Here's how the part is built. I have some questions about the finished solid (model axes, mm). Face numbers are marked on the shaded views. A direction names the side the tool comes from. Round coordinates to 2 decimals unless told otherwise and drop trailing zeros. Order: outer loops, then holes, each group sorted by start corner. A loop starts at its lowest first (then second) coordinate and runs counter-clockwise, first axis right, second up. Notation, with made-up numbers: (66.5, 63.25) -> (107.5, 63.25) arc R26 ccw to (107.5, 101.25) -> close; hole circle Ø4 at (24, 47.5). An arc over 180 degrees is marked (long way). Answer in a Markdown table with one row per item.
Autodesk Inventor part; units mm, degrees
ref_plane "Płaszczyzna konstrukcyjna1" through (0, 0, 8) normal (0, 0, -1) x (-1, 0, 0)
ref_plane "YZ Plane" through (0, 0, 0) normal (1, 0, 0) x (0, 1, 0)
ref_plane "XZ Plane" through (0, 0, 0) normal (0, 1, 0) x (-1, 0, 0)
sketch "Szkic1" plane through (0, 0, 0) normal (0, 0, 1) x (1, 0, 0)
  line L0 (-14, 0) -> (14, 0)
  line L1 (0, -14) -> (0, 14)
  circle A0 centre (0, 0) radius 10
  circle A1 centre (0, 0) radius 1.8
  line L2 (-1.3416, 1.2) -> (1.3416, 1.2)
  dimension "d1" = 20
  dimension "d2" = 3.6
  dimension "d3" = 1.2
extrude "Wyciągnięcie proste1" add sketch "Szkic1" along normal blind 20 contours A1 L1 A0 L0 | L0 A0 L1 A1 | L2 L1 A1 | L1 A0 L0 A1 | L1 A1 L0 A0 | L2 A1 L1
ref_plane "Płaszczyzna konstrukcyjna1" through (0, 0, 8) normal (0, 0, -1) x (-1, 0, 0)
sketch "Szkic2" plane through (0, 0, 8) normal (0, 0, -1) x (-1, 0, 0)
  circle A0 centre (0, 0) radius 10
  arc A1 (-1.3416, 1.2) -> (1.3416, 1.2) centre (0, 0) ccw
  line L0 (1.3416, 1.2) -> (-1.3416, 1.2)
  circle A2 centre (0, 0) radius 12
  dimension "d7" = 24
extrude "Wyciągnięcie proste2" add sketch "Szkic2" against normal blind 4 contours A2
sketch "Szkic3" plane through (0, 0, 0) normal (0, 0, -1) x (-1, 0, 0)
  circle A0 centre (0, 0) radius 10
  arc A1 (-1.3416, 1.2) -> (1.3416, 1.2) centre (0, 0) ccw
  line L0 (1.3416, 1.2) -> (-1.3416, 1.2)
  circle A2 centre (0, 0) radius 12
  circle A3 centre (0, 0) radius 10
  line L1 (16.8, 0) -> (-16.8, 0)
  line L2 (0, -16.8) -> (0, 16.8)
  line L3 (2, -11) -> (-2, -11)
  line L4 (-2, -11) -> (-2, -9)
  line L5 (-2, -9) -> (2, -9)
  line L6 (2, -9) -> (2, -11)
  circle A4 centre (0, 0) radius 10
  line L7 (2, -11) -> (-2, -9) construction
  line L8 (-2, -11) -> (2, -9) construction
  point P0 (0, -10)
  dimension "d11" = 4
  dimension "d12" = 2
extrude "Wyciągnięcie proste3" cut sketch "Szkic3" against normal up to surface (20 mm away) contours L6 L3 L2 A0 | A0 L2 L5 L6 | L2 L3 L4 A0 | A0 L4 L5 L2
pattern_circular "Szyk kołowy1" count 6 over 360 about axis through (0, 0, -10) along (0, 0, 1) of "Wyciągnięcie proste3"
sketch "Szkic4" plane through (0, 0, 20) normal (0, 0, 1) x (1, 0, 0)
  circle A0 centre (0, 0) radius 14
  circle A1 centre (0, 0) radius 8.25
  dimension "d20" = 28
  dimension "d21" = 16.5
extrude "Wyciągnięcie proste4" cut sketch "Szkic4" against normal blind 10 contours A1
properties part number "koło" material "Tworzywo sztuczne PET"
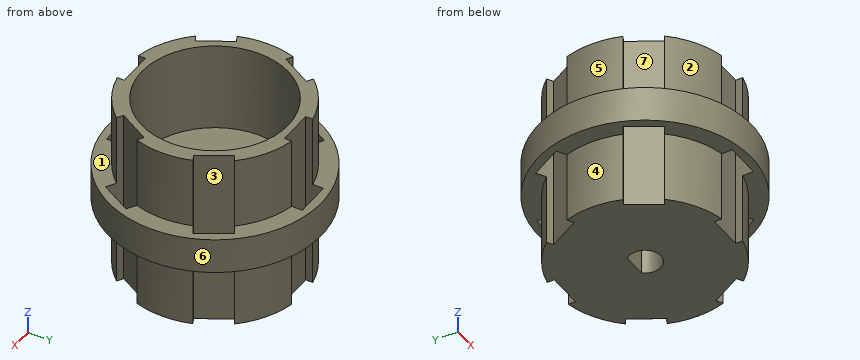
1. Suppose I cut it at B-B on x = 0. Write out the boundary of the cut face in (y, z), then the cut area to 3 significant figures.
Numbers:
| item | result |
|---|---|
| outline | (-12, 8) -> (-11, 8) -> (-11, 12) -> (-12, 12) -> close; (-9, 0) -> (-1.8, 0) -> (-1.8, 10) -> (-8.25, 10) -> (-8.25, 20) -> (-9, 20) -> close; (1.2, 0) -> (9, 0) -> (9, 20) -> (8.25, 20) -> (8.25, 10) -> (1.2, 10) -> close; (11, 8) -> (12, 8) -> (12, 12) -> (11, 12) -> close |
| area | 173 mm2 |
2. We'd pull the mould along X, two halves only. Please class the marked faces 5, 6 and 7: released by +X, released by -X, zero draft, split by the parting line, or undercut.
Numbers:
| item | result |
|---|---|
| face 5 | released by -X |
| face 6 | split by the parting line |
| face 7 | undercut |
3. Please list where these lines run through material, in increasing order: line 1 along Y through (x, z) = (0, 2.5); line 2 along X through (y, z) = (-5, 10.5); line 3 along Y through (x, z) = (0, 17).
Numbers:
| item | result |
|---|---|
| line 1 | y = -9 to -1.8, 1.2 to 9 |
| line 2 | x = -10.91 to -9.81, -7.51 to -6.56, 6.56 to 7.51, 9.81 to 10.91 |
| line 3 | y = -9 to -8.25, 8.25 to 9 |
4. For pin 1 Ø2 at (x, z) = (-0.5, 5.5) entering from -Y; pin 2 Ø5 at (x, y) = (-2, 3) entering from +Z; pin 3 Ø2 at (y, z) = (-10, 6) entering from +X; pin 4 Ø0.6 at (y, z) = (10.5, 13) entering from +X, each with a flat end and sliding along its axis, tell me the tip position at first contact or that it passes through.
Numbers:
| item | result |
|---|---|
| pin 1 | stops at y = -9 |
| pin 2 | stops at z = 10 |
| pin 3 | stops at x = 4.36 |
| pin 4 | passes through |
5. For the marked faces 1, 2, 3 and 4, which set-ups out of +Z, -Z, +X, -X, +Y, -Y let a thin tool reach every point of the face, with its end or its side?
Numbers:
| item | result |
|---|---|
| face 1 | +Z |
| face 2 | +Z, -X, -Y |
| face 3 | +Z, -Z |
| face 4 | -Z, -X |
6. Suppose I cut it at C-C on z = 9.5. Write out the boundary of the cut face in (x, y), then the cut area to 3 significant figures.
Numbers:
| item | result |
|---|---|
| outline | circle Ø24 at (0, 0); hole (-10.53, -3.77) -> (-8.53, -7.23) -> (-6.79, -6.23) -> (-8.79, -2.77) -> close; hole (-10.53, 3.77) -> (-8.79, 2.77) -> (-6.79, 6.23) -> (-8.53, 7.23) -> close; hole (-2, -11) -> (2, -11) -> (2, -9) -> (-2, -9) -> close; hole (-2, 9) -> (2, 9) -> (2, 11) -> (-2, 11) -> close; hole (-1.34, 1.2) arc R1.8 ccw (long way) to (1.34, 1.2) -> close; hole (6.79, -6.23) -> (8.53, -7.23) -> (10.53, -3.77) -> (8.79, -2.77) -> close; hole (6.79, 6.23) -> (8.79, 2.77) -> (10.53, 3.77) -> (8.53, 7.23) -> close |
| area | 395 mm2 |
7. Suppose I cut it at D-D on y = 10.25. Write out the boundary of the cut face in (x, z), then the cut area to 3 significant figures.
Numbers:
| item | result |
|---|---|
| outline | (-6.24, 8) -> (-2, 8) -> (-2, 12) -> (-6.24, 12) -> close; (2, 8) -> (6.24, 8) -> (6.24, 12) -> (2, 12) -> close |
| area | 33.9 mm2 |
8. Suppose I cut it at A-A on y = 0. Write out the boundary of the cut face in (x, z), then the cut area to 3 significant figures.
Numbers:
| item | result |
|---|---|
| outline | (-12, 8) -> (-10, 8) -> (-10, 0) -> (-1.8, 0) -> (-1.8, 10) -> (-8.25, 10) -> (-8.25, 20) -> (-10, 20) -> (-10, 12) -> (-12, 12) -> close; (1.8, 0) -> (10, 0) -> (10, 8) -> (12, 8) -> (12, 12) -> (10, 12) -> (10, 20) -> (8.25, 20) -> (8.25, 10) -> (1.8, 10) -> close |
| area | 215 mm2 |
